Design review of the part built by this model. Coordinates are the model's own, in mm. Face numbers are marked on the shaded views. Coordinates: 2 decimals unless noted, no trailing zeros. Write each loop counter-clockwise with the first axis right and the second up, starting at its lowest first coordinate (ties: lowest second). Pieces come first, ordered by that corner, then holes. Notation, with made-up numbers: M 6.25,-34 L 23.25,-34 A17 ccw 23.25,-30 Z; hole C 44.5,36.5 d6. An arc over 180 degrees is marked long. Return JSON: item names as keys, results as strings. Group by question number.
```python
from build123d import *

# Parameters (mm, degrees)
SKETCH1_R           = 12.5
SKETCH1_R_2         = 0.5
BOSS_EXTRUDE1_DEPTH = 6.35
SKETCH2_W           = 4.35
SKETCH2_H           = 4.5


with BuildPart() as part:
    # Sketch1 → Boss-Extrude1 (new body)
    with BuildSketch(Plane.XY):
        Circle(SKETCH1_R)
        Circle(SKETCH1_R_2, mode=Mode.SUBTRACT)
    extrude(amount=BOSS_EXTRUDE1_DEPTH)

    # Sketch2 → Cut-Revolve1 (revolve, cut)
    with BuildSketch(Plane(origin=(0, 0, 0), x_dir=(0, 0, -1), z_dir=(1, 0, 0))):
        with Locations((-3.175, 10.25)):
            Rectangle(SKETCH2_W, SKETCH2_H)
    revolve(axis=Axis((0, 0, 0), (0, 0, 1)), mode=Mode.SUBTRACT)


solid = part.part
```
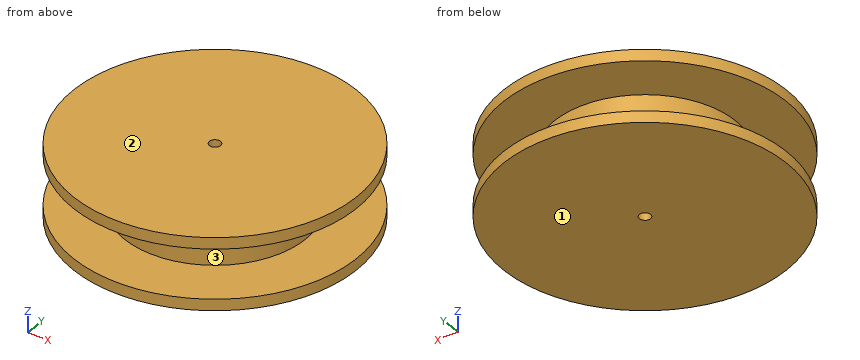
Item 1: The part is to be moulded in two halves that separate along Z. For the marked faces 1, 2 and 3, say which applies: pulls with the +Z half, pulls with the -Z half, needs draft (parallel to the pull), parting line crosses it, or undercut.
Item 2: For line 1 (Y direction, x = 0, z = 3.5); line 2 (Z direction, x = -5.25, y = -6.75); line 3 (Y direction, x = -2.75, z = 3.25), list the stretches that pass through material, from the lowest coordinate up.
Item 3: Add section D-D (y = -7.5). Write out the cut boundary in (x, z), plus the area to 3 significant figures.
Item 4: Add section A-A (x = 0). Write out the cut boundary in (y, z), plus the area to 3 significant figures.
Item 5: Add section C-C (z = 2.25). Write out the cut boundary in (x, y).
Item 6: For pin 1 (1.5 mm diameter, centred on x = 4, z = 4.5, fed in from +Y); pin 2 (1.5 mm diameter, centred on x = 5.5, z = 4, fed in from -Y), all flat-tipped, find the tip position at first contact; note any pin that passes through.
Geometry check:
{
 "1": {"face 1": "pulls with the -Z half", "face 2": "pulls with the +Z half", "face 3": "undercut"},
 "2": {"line 1": "-8 to -0.5, 0.5 to 8", "line 2": "0 to 1, 5.35 to 6.35", "line 3": "-7.51 to 7.51"},
 "3": {"outline": "M -10,0 L 10,0 L 10,1 L 2.78,1 L 2.78,5.35 L 10,5.35 L 10,6.35 L -10,6.35 L -10,5.35 L -2.78,5.35 L -2.78,1 L -10,1 Z", "area": "64.2 mm^2"},
 "4": {"outline": "M -12.5,0 L -0.5,0 L -0.5,6.35 L -12.5,6.35 L -12.5,5.35 L -8,5.35 L -8,1 L -12.5,1 Z; M 0.5,0 L 12.5,0 L 12.5,1 L 8,1 L 8,5.35 L 12.5,5.35 L 12.5,6.35 L 0.5,6.35 Z", "area": "113 mm^2"},
 "5": {"outline": "C 0,0 d16; hole C 0,0 d1"},
 "6": {"pin 1": "y = 7.31", "pin 2": "y = -6.44"}
}
